CAD build for the part. Positions are in the model's coordinates, mm. Face numbers are marked on the shaded views. A direction names the side the tool comes from. Coordinates: 2 decimals unless noted, no trailing zeros. Loops run counter-clockwise (first coordinate to the right, second up) from the corner with the lowest first, then second, coordinate; pieces in that order, holes last. Notation, with made-up numbers: (44, -11) -> (71, -11) arc R20 cw to (71, -7) -> close; hole circle Ø8 at (11, 4.5). An arc over 180 degrees is marked (long way). Return JSON: item names as keys, results as strings. Group by question number.
(1) Saw through at A-A on x = -16.75. Write the cut outline in (y, z).
(2) Saw through at D-D on z = 11. Write the cut outline in (x, y).
(3) Saw through at B-B on z = 3. Write the cut outline in (x, y).
(4) Saw through at C-C on y = 3.75. Write the cut outline in (x, z), then the cut area to 3 significant figures.
(5) Tool access for the marked faces 1, 2 and 3: list every direction of +Z, -Z, +X, -X, +Y, -Y with a clear straight run to the whole face (end or side of a thin tool).
(6) Flat gauge pins, fed straight in: pin 1 Ø1.2 at (x, z) = (-30.5, 13.5) entering from -Y; pin 2 Ø4 at (x, y) = (-19, -6) entering from +Z; pin 3 Ø1.1 at (x, z) = (-23, 14) entering from -Y. Where does each tip first touch, or does it go through?
(7) Probe L1, parallel to Z at x = -28.75, y = 0.25; L2, parallel to X at y = 10, z = 11.75; L3, parallel to Y at x = -29.5, z = 2.5. List the from-to ranges inside material, lowest first.
(8) Mould opens along X. For the marked faces 4, 5, 6 and 7 say: pulls with the +X half, pulls with the -X half, needs draft (parallel to the pull), parting line crosses it, or undercut.
```python
from build123d import *

# Parameters (mm, degrees)
CROQUIS1_W              = 19
CROQUIS1_H              = 29
SALIENTE_EXTRUIR1_DEPTH = 6
SALIENTE_EXTRUIR2_DEPTH = 4.5
CROQUIS3_W              = 19
CROQUIS3_H              = 11.5
SALIENTE_EXTRUIR3_DEPTH = 1.5
CROQUIS4_W              = 12
CROQUIS4_H              = 4
CORTAR_EXTRUIR1_DEPTH   = 5
SALIENTE_EXTRUIR4_DEPTH = 7.5
SALIENTE_EXTRUIR5_DEPTH = 1
CORTAR_EXTRUIR2_START   = -19
CROQUIS7_W              = 3
CROQUIS7_H              = 22
CORTAR_EXTRUIR2_DEPTH   = 19


with BuildPart() as part:
    # Croquis1 → Saliente-Extruir1 (new body)
    with BuildSketch(Plane.XY):
        with Locations((-22.223018523, 5.939759036)):
            Rectangle(CROQUIS1_W, CROQUIS1_H)
    extrude(amount=SALIENTE_EXTRUIR1_DEPTH)

    # Croquis2 → Saliente-Extruir2 (add)
    with BuildSketch(Plane.XY.offset(6)):
        Polygon((-31.723018523, -8.560240964), (-31.723018523, 2.939759036), (-30.223018523, 2.939759036), (-30.223018523, -7.060240964), (-14.223018523, -7.060240964), (-14.223018523, 2.939759036), (-12.723018523, 2.939759036), (-12.723018523, -8.560240964), align=None)
    extrude(amount=SALIENTE_EXTRUIR2_DEPTH)

    # Croquis3 → Saliente-Extruir3 (add)
    with BuildSketch(Plane.XY.offset(10.5)):
        with Locations((-22.223018523, -2.810240964)):
            Rectangle(CROQUIS3_W, CROQUIS3_H)
    extrude(amount=SALIENTE_EXTRUIR3_DEPTH)

    # Croquis4 → Cortar-Extruir1 (cut)
    with BuildSketch(Plane.XZ.offset(8.560240964)):
        with Locations((-21.223018523, 7.3)):
            Rectangle(CROQUIS4_W, CROQUIS4_H)
    extrude(amount=-CORTAR_EXTRUIR1_DEPTH, mode=Mode.SUBTRACT)

    # Croquis5 → Saliente-Extruir4 (add)
    with BuildSketch(Plane.XY.offset(6)):
        Polygon((-30.223018523, 2.939759036), (-31.723018523, 2.939759036), (-31.723018523, 20.439759036), (-12.723018523, 20.439759036), (-12.723018523, 2.939759036), (-14.223018523, 2.939759036), (-14.223018523, 18.939759036), (-30.223018523, 18.939759036), align=None)
    extrude(amount=SALIENTE_EXTRUIR4_DEPTH)

    # Croquis6 → Saliente-Extruir5 (add)
    with BuildSketch(Plane.XY.offset(13.5)):
        Polygon((-29.223018523, 2.939759036), (-31.723018523, 2.939759036), (-31.723018523, 20.439759036), (-12.723018523, 20.439759036), (-12.723018523, 2.939759036), (-15.223018523, 2.939759036), (-15.223018523, 17.939759036), (-29.223018523, 17.939759036), align=None)
    extrude(amount=SALIENTE_EXTRUIR5_DEPTH)

    # Croquis7 → Cortar-Extruir2 (cut)
    with BuildSketch(Plane(origin=(-12.723018523, 0, 0), x_dir=(0, 0, -1), z_dir=(1, 0, 0)).offset(CORTAR_EXTRUIR2_START)):
        with Locations((-3, 5.939759036)):
            Rectangle(CROQUIS7_W, CROQUIS7_H)
    extrude(amount=CORTAR_EXTRUIR2_DEPTH, mode=Mode.SUBTRACT)


solid = part.part
```
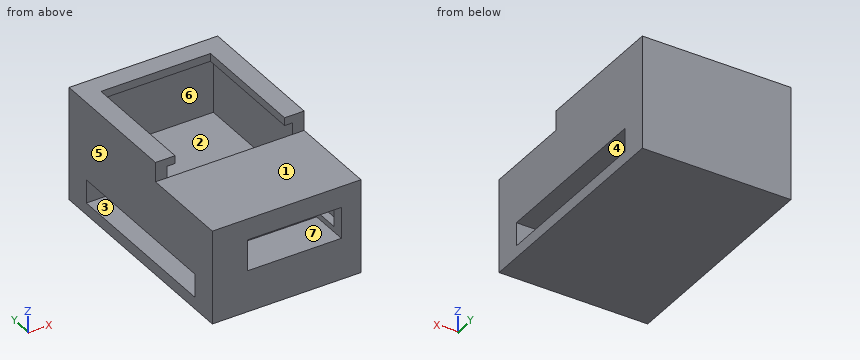
Geometry results:
{
 "1": {"outline": "(-8.56, 0) -> (20.44, 0) -> (20.44, 14.5) -> (17.94, 14.5) -> (17.94, 13.5) -> (18.94, 13.5) -> (18.94, 6) -> (-3.56, 6) -> (-3.56, 5.3) -> (-8.56, 5.3) -> close; (-8.56, 9.3) -> (-7.06, 9.3) -> (-7.06, 10.5) -> (2.94, 10.5) -> (2.94, 12) -> (-8.56, 12) -> close; hole (-5.06, 1.5) -> (16.94, 1.5) -> (16.94, 4.5) -> (-5.06, 4.5) -> close"},
 "2": {"outline": "(-31.72, -8.56) -> (-12.72, -8.56) -> (-12.72, 20.44) -> (-31.72, 20.44) -> close; hole (-30.22, 2.94) -> (-14.22, 2.94) -> (-14.22, 18.94) -> (-30.22, 18.94) -> close"},
 "3": {"outline": "(-31.72, -8.56) -> (-12.72, -8.56) -> (-12.72, -5.06) -> (-31.72, -5.06) -> close; (-31.72, 16.94) -> (-12.72, 16.94) -> (-12.72, 20.44) -> (-31.72, 20.44) -> close"},
 "4": {"outline": "(-31.72, 0) -> (-12.72, 0) -> (-12.72, 1.5) -> (-31.72, 1.5) -> close; (-31.72, 4.5) -> (-12.72, 4.5) -> (-12.72, 14.5) -> (-15.22, 14.5) -> (-15.22, 13.5) -> (-14.22, 13.5) -> (-14.22, 6) -> (-30.22, 6) -> (-30.22, 13.5) -> (-29.22, 13.5) -> (-29.22, 14.5) -> (-31.72, 14.5) -> close", "area": "84.5 mm²"},
 "5": {"face 1": "+Z, +X, -X, -Y", "face 2": "none", "face 3": "+X, -X"},
 "6": {"pin 1": "y = 2.94", "pin 2": "z = 12", "pin 3": "y = 17.94"},
 "7": {"L1": "0 to 1.5, 4.5 to 6, 10.5 to 12", "L2": "-31.72 to -30.22, -14.22 to -12.72", "L3": "-8.56 to -5.06, 16.94 to 20.44"},
 "8": {"face 4": "needs draft", "face 5": "pulls with the -X half", "face 6": "undercut", "face 7": "undercut"}
}
